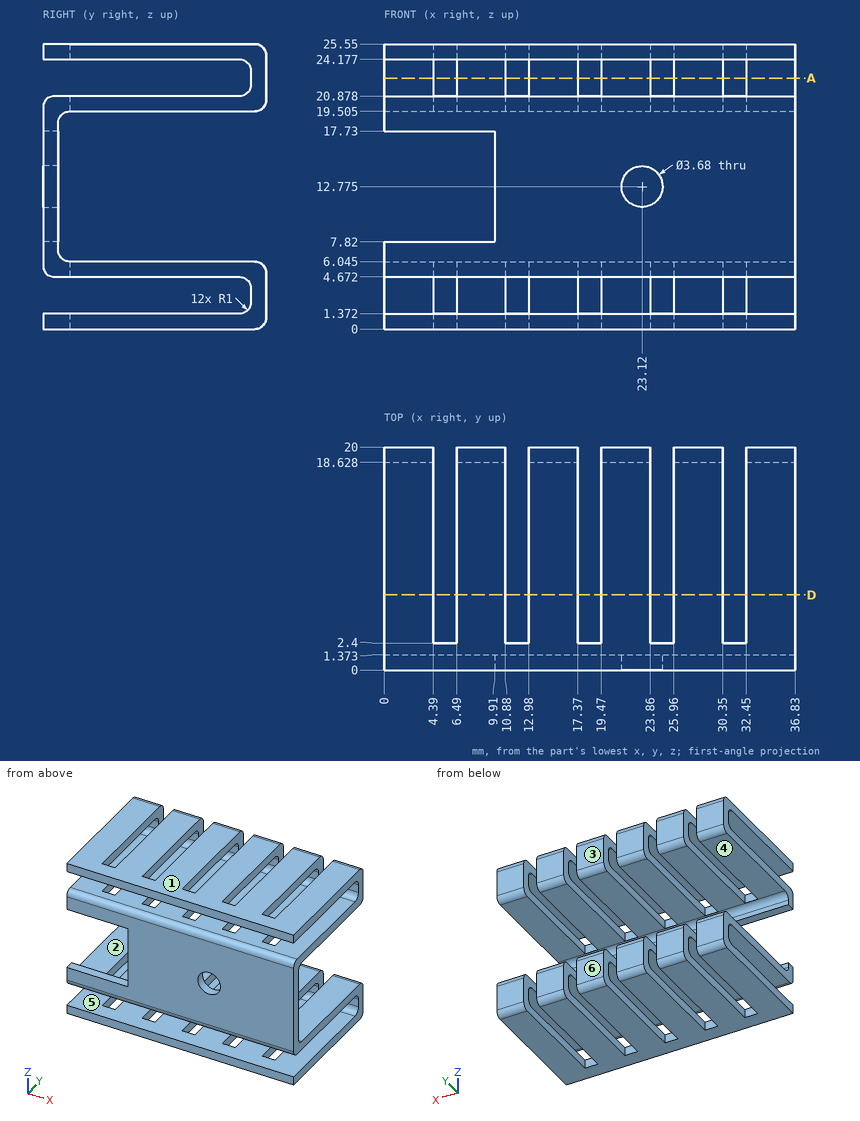
Can you work these out from the drawing? Everything is in mm from the part's minimum corner. A direction names the side the tool comes from. Round coordinates to 2 decimals unless told otherwise and drop trailing zeros. Order: outer loops, then holes, each group sorted by start corner. A loop starts at its lowest first (then second) coordinate and runs counter-clockwise, first axis right, second up. Notation, with made-up numbers: M -22,-12 L 29,-12 A14 ccw 29,5 Z; hole C -26.5,1 d4. An arc over 180 degrees is marked long. Answer as CSV lines item,"result".
Item 1: We'd pull the mould along Z, two halves only. Please class the marked faces 1, 2 and 3: +Z half, -Z half, draft (parallel to the pull), parting line (faces both ways), or undercut.
From the geometry:
face 1,"+Z half"
face 2,"undercut"
face 3,"draft"
Item 2: Imagine slicing it at A-A on z = 22.5. List the corners of the cut face in (x, y) for me.
From the geometry:
outline,"M 0,18.63 L 4.39,18.63 L 4.39,20 L 0,20 Z; M 6.49,18.63 L 10.88,18.63 L 10.88,20 L 6.49,20 Z; M 12.98,18.63 L 17.37,18.63 L 17.37,20 L 12.98,20 Z; M 19.47,18.63 L 23.86,18.63 L 23.86,20 L 19.47,20 Z; M 25.96,18.63 L 30.35,18.63 L 30.35,20 L 25.96,20 Z; M 32.45,18.63 L 36.83,18.63 L 36.83,20 L 32.45,20 Z"
Item 3: Which directions (+Z, -Z, +X, -X, +Y, -Y) give clear straight access to the entire face, cutting with the end or side of a thin tool? Please do the marked faces 4, 5 and 6.
From the geometry:
face 4,"+X, -X, +Y"
face 5,"+X, -X, -Y"
face 6,"+Z, -Z, +X, -X, +Y"
Item 4: Imagine slicing it at D-D on y = 6.75. Give the number of separate pieces and of enclosed holes in the cut face.
From the geometry:
separate pieces,"24"
enclosed holes,"0"
Item 5: Please list where these lines run through material, in increasing order: L1, parallel to X at y = 8.25, z = 5.25; L2, parallel to Y at x = 29, z = 9; L3, parallel to Y at x = 28, z = 22. Write a range as [from, to].
From the geometry:
L1,"[0, 4.39], [6.49, 10.88], [12.98, 17.37], [19.47, 23.86], [25.96, 30.35], [32.45, 36.83]"
L2,"[0, 1.37]"
L3,"[18.63, 20]"
Item 6: For pin 1 (0.6 mm diameter, centred on x = 21, z = 3.5, fed in from -Y); pin 2 (1.1 mm diameter, centred on x = 19, z = 0.5, fed in from +Y); pin 3 (0.7 mm diameter, centred on x = 31.5, z = 0.5, fed in from +Y), each with a flat end and sliding along its axis, tell me the tip position at first contact or that it passes through.
From the geometry:
pin 1,"y = 18.62"
pin 2,"y = 19.98"
pin 3,"y = 2.4"
